For this review, take the finished solid that the model builds, in its own axes (mm). Give positions to 0.01 mm unless a question says otherwise; leave off trailing zeros. Loops run counter-clockwise (first coordinate to the right, second up) from the corner with the lowest first, then second, coordinate; pieces in that order, holes last. Notation, with made-up numbers: (10.25, -23) - (59.25, -23) arc R16 ccw to (59.25, 3) - close; hole circle Ø7 at (43.5, 8). An arc over 180 degrees is marked (long way). Put each result on its own line as item: value. Start each with the question number.
Autodesk Inventor part; units mm, degrees
ref_plane "YZ Plane" through (0, 0, 0) normal (1, 0, 0) x (0, 1, 0)
ref_plane "XZ Plane" through (0, 0, 0) normal (0, 1, 0) x (-1, 0, 0)
ref_plane "XY Plane" through (0, 0, 0) normal (0, 0, 1) x (1, 0, 0)
sketch "Skizze1" plane through (0, 0, 0) normal (0, 1, 0) x (-1, 0, 0)
  line L0 (0, 42.9058) -> (-350, 42.9058)
  line L1 (-350, 42.9058) -> (-350, -17.0942)
  line L2 (-350, -17.0942) -> (0, -17.0942)
  line L3 (0, -17.0942) -> (0, 42.9058)
  point P0 (0, 0)
  dimension "d0" = 350
  dimension "d1" = 0
  dimension "d2" = 60
extrude "Extrusion1" add sketch "Skizze1" along normal blind 10
sketch "Skizze2" plane through (0, 10, 0) normal (0, 1, 0) x (1, 0, 0)
  line L0 (25, 0.0942) -> (325, 0.0942)
  line L1 (325, 0.0942) -> (325, -25.9058)
  line L2 (325, -25.9058) -> (25, -25.9058)
  line L3 (25, -25.9058) -> (25, 0.0942)
  line L4 (0, 17.0942) -> (0, -42.9058)
  line L5 (350, -42.9058) -> (350, 17.0942)
  line L6 (350, 17.0942) -> (0, 17.0942)
  line L7 (0, -42.9058) -> (350, -42.9058)
  point P0 (0, 0)
  point P1 (175, 17.0942)
  dimension "d5" = 25
  dimension "d6" = 25
  dimension "d7" = 17
  dimension "d8" = 17
extrude "Extrusion2" cut sketch "Skizze2" against normal through all contours L0 L1 L2 L3
fillet "Rundung1" radius 2 1 edges at (25, 5, -0.0942)
fillet "Rundung2" radius 2 1 edges at (25, 5, 25.9058)
fillet "Rundung3" radius 2 1 edges at (325, 5, -0.0942)
fillet "Rundung4" radius 2 1 edges at (325, 5, 25.9058)
sketch "Skizze4" plane through (0, 10, 0) normal (0, 1, 0) x (1, 0, 0)
  line L0 (20, -30.9058) -> (330, -30.9058)
  line L1 (330, 5.0942) -> (20, 5.0942)
  line L2 (25, -23.9058) -> (25, -1.9058)
  line L3 (323, -25.9058) -> (27, -25.9058)
  line L4 (27, 0.0942) -> (323, 0.0942)
  line L5 (325, -1.9058) -> (325, -23.9058)
  arc A0 (20, 5.0942) -> (20, 0.0942) centre (20, 2.5942) ccw
  arc A1 (20, -25.9058) -> (20, -30.9058) centre (20, -28.4058) ccw
  arc A2 (330, 0.0942) -> (330, 5.0942) centre (330, 2.5942) ccw
  arc A3 (330, -30.9058) -> (330, -25.9058) centre (330, -28.4058) ccw
  line L6 (330, 0.0942) -> (330, -25.9058)
  line L7 (20, 0.0942) -> (20, -25.9058)
  point P0 (0, 0)
  dimension "d32" = 5
  dimension "d33" = 5
  dimension "d110" = 2.5
  dimension "d111" = 2.5
  dimension "d112" = 2.5
  dimension "d113" = 2.5
  dimension "d114" = 5
  dimension "d115" = 5
extrude "Extrusion4" cut sketch "Skizze4" against normal blind 8
sketch "Skizze14" plane through (0, 0, 0) normal (0, -1, 0) x (1, 0, 0)
  line L0 (0, 42.9058) -> (350, 42.9058)
  line L1 (0, -17.0942) -> (0, 42.9058)
  point P0 (0, 0)
  point P1 (16.3, 39.1558)
  dimension "d116" = 3.75
  dimension "d117" = 16.3
hole "Bohrung8" at (16.3, 0, 39.1558) direction (0, 1, 0) diameter 3.4 end through all counterbore diameter 6.5 counterbore depth 3.4
pattern_linear "Rechteckige Anordnung2" count 14 spacing 24.6 along (1, 0, 0) count 2 spacing 52.5 along (0, 0, -1) of "Bohrung8"
equation "\"d32\" = d33"
equation "\"d114\" = d33"
equation "\"d115\" = d33"
1) Mouldability with a two-part tool opening along Z and no side actions: class faces 1 (the cylindrical face through (209.878, 1.724, -12.921)), 2 (the flat face through (330, 6, 13)) as released by +Z, released by -Z, zero draft, split by the parting line, or undercut.
2) Take a section at A-A on x = 181.5. State the section outline as (y, z) points, and give its area (3 significant figures).
3) Wall thickness on probe 1 along Z at (x, y) = (311.5, 0.9); probe 2 along Z at (x, y) = (65.5, 2.4); probe 3 along X at (y, z) = (9.5, 11.5): over which ranges is each line inside the solid? List them lowest first.
4) Insertion check: P1, Ø3, axis at x = 213.1, z = 39.16, coming from the +Y side (3 decimals); P2, Ø10, axis at x = 192.5, z = 2, coming from the +Y side; P3, Ø3, axis at x = 40.5, z = -14, coming from the -Y side. Each pin has a flat end and moves straight along its axis. Give the tip position at first contact, or say it passes through.
Answers follow:
1. face 1: undercut
1. face 2: undercut
2. outline: (0, -17.09) - (10, -17.09) - (10, -5.09) - (2, -5.09) - (2, -0.09) - (0, -0.09) - close; (0, 25.91) - (2, 25.91) - (2, 30.91) - (10, 30.91) - (10, 42.91) - (0, 42.91) - close
2. area: 260 mm2
3. probe 1: -17.09 to -16.59, -10.09 to -0.09, 25.91 to 35.91, 42.41 to 42.91
3. probe 2: -17.09 to -16.59, -10.09 to -5.09, 30.91 to 35.91, 42.41 to 42.91
3. probe 3: 0 to 20, 330 to 350
4. P1: through
4. P2: y = 2
4. P3: y = 3.4
